Source: three-view drawing plus pictorial views. Frame: mm from the lowest corner of the part. A direction names the side the tool comes from. Coordinates: 2 decimals unless noted, no trailing zeros. Answer as a JSON object with one key per item and string values. Group by question number.
Item 1: Line query: line 1 along Z through (x, y) = (124, 22.75) (1 decimal); line 2 along X through (y, z) = (6.75, 39.5); line 3 along Y through (x, z) = (71.5, 126.5). Output: solid intervals per line, ascending. Write a range as from..to.
Item 2: Mould query, pull axis Z, two halves, no side actions, for the marked faces 4, 5 and 6. Classes: pulls with the +Z half, pulls with the -Z half, needs draft (parallel to the pull), parting line crosses it, or undercut.
Item 3: First-contact query: pin 1 Ø6 at (y, z) = (5, 124.5) entering from -X; pin 2 Ø4 at (x, z) = (31.5, 39.5) entering from -Y; pin 3 Ø10 at (y, z) = (10, 64.5) entering from -X. Flat tips, straight axial feed; report the tip coordinate or a pass-through.
Item 4: Set-up query: the marked faces 1, 2 and 3. Return all of +Z, -Z, +X, -X, +Y, -Y with unobstructed straight access to the full face (end or side cutting, diameter ignored); none if empty.
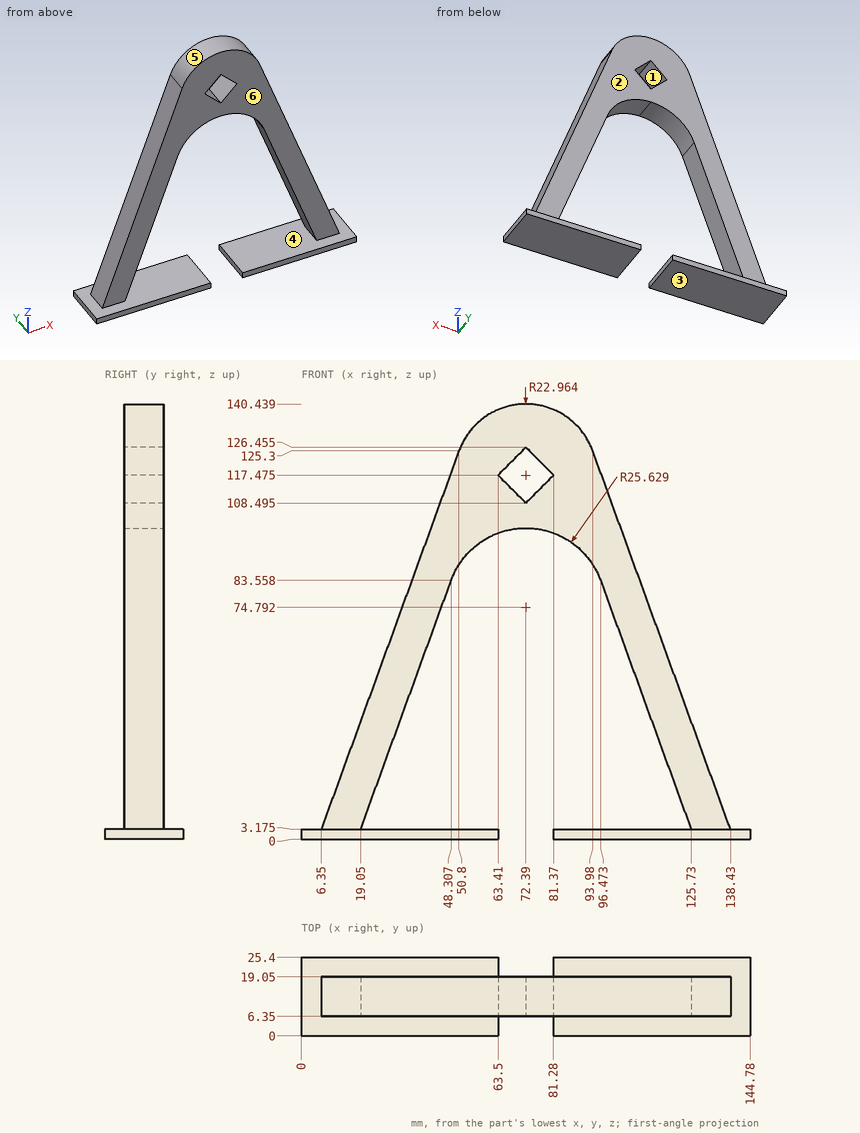
Checks:
{
 "1": {"line 1": "0..3.2", "line 2": "19.57..32.27, 112.51..125.21", "line 3": "6.35..19.05"},
 "2": {"face 4": "undercut", "face 5": "pulls with the +Z half", "face 6": "needs draft"},
 "3": {"pin 1": "x = 49.53", "pin 2": "y = 6.35", "pin 3": "x = 26.85"},
 "4": {"face 1": "+Y, -Y", "face 2": "+Z, +X, -X, +Y", "face 3": "-Z, +X, -X, +Y, -Y"}
}
